For this review, take the finished solid that the model builds, in its own axes (mm). Coordinates: 2 decimals unless noted, no trailing zeros. Write each loop counter-clockwise with the first axis right and the second up, starting at its lowest first coordinate (ties: lowest second). Pieces come first, ordered by that corner, then holes. Notation, with made-up numbers: (58, 25.5) -> (115, 25.5) arc R19 ccw to (115, 33.5) -> close; hole circle Ø9 at (34.25, 0.5). An arc over 180 degrees is marked (long way). One line per item, written item: value. Start each with the question number.
1) For probe 1 along Z at (x, y) = (-9.6, -24.5); probe 2 along Y at (x, z) = (-9.4, 8.5); probe 3 along Y at (x, z) = (-10.65, 10), list the stretches that pass through material, from the lowest coordinate up. Write a range as from..to.
2) Add section C-C (z = 20). State the section outline as (x, y) points, and give its area (3 significant figures).
3) For pin 1 Ø1.5 at (y, z) = (-31, 32.5) entering from +X; pin 2 Ø1 at (x, z) = (-10, 32.5) entering from -Y; pin 3 Ø1 at (x, y) = (-10, -31.5) entering from +Z, all flat-tipped, find the tip position at first contact; note any pin that passes through.
4) Add section A-A (x = -10.1). State the section outline as (y, z) points.
5) Add section B-B (y = -66.5). State the section outline as (x, z) points, and give its area (3 significant figures).
Autodesk Inventor part; units mm, degrees
ref_plane "YZ Plane" through (0, 0, 0) normal (1, 0, 0) x (0, 1, 0)
ref_plane "XZ Plane" through (0, 0, 0) normal (0, 1, 0) x (-1, 0, 0)
ref_plane "XY Plane" through (0, 0, 0) normal (0, 0, 1) x (1, 0, 0)
ref_plane "Work Plane4" through (-12.2663, 34.5, -3) normal (-1, 0, 0) x (0, 0, 1)
sketch "Sketch4" plane through (-12.2663, 34.5, -3) normal (-1, 0, 0) x (0, 0, 1)
  line L0 (0, 0) -> (0, -108)
  line L1 (0, -108) -> (3, -108)
  line L2 (3, 0) -> (3, -108)
  line L3 (0, 0) -> (3, 0)
  circle A0 centre (13.5, 27.5) radius 25
  line L4 (7.5, -120) -> (3, -120)
  line L5 (3, -120) -> (3, -124)
  line L6 (3, -124) -> (-0.5, -124)
  line L7 (-0.5, -124) -> (-0.5, -138)
  line L8 (-0.5, -138) -> (8.5, -124)
  line L9 (8.5, -124) -> (7.5, -124)
  line L10 (7.5, -124) -> (7.5, -120)
  line L11 (0, -111) -> (3, -111)
  line L12 (0, -111) -> (0, -124)
  line L13 (0, -124) -> (3, -124)
  line L14 (3, -111) -> (3, -124)
  line L15 (3, -111) -> (3, -108)
  line L16 (0, -108) -> (0, -111)
  line L17 (7.5, -120) -> (3, -120)
  line L18 (3, -120) -> (3, 0)
  line L19 (3, 0) -> (36.5, 0)
  line L20 (8.5, -124) -> (66.1149, -34.3768)
  line L21 (7.5, -120) -> (63.7229, -32.5421)
  line L22 (36.5, 0) -> (36.5, -74.8889)
  line L23 (36.5, -72.0889) -> (33.5, -72.0889)
  line L24 (33.5, -72.0889) -> (33.5, -56.9889)
  line L25 (33.5, -56.9889) -> (36.5, -56.9889)
  line L26 (36.5, -56.9889) -> (36.5, -72.0889)
  point P0 (3, -34.5)
  point P1 (38.5, 27.5)
  point P2 (36.5, -56.9889)
  dimension "d4" = 25
  dimension "d5" = 2
  dimension "d9" = 2.8
  dimension "d10" = 15.1
  dimension "d11" = 3
extrude "Extrusion1" add sketch "Sketch4" against normal blind 3 contours L19 L22 L25 L24 L23 L21 L4 L14 L15 L2
sketch "Sketch8" plane through (-12.2663, -37.5889, 30.5) normal (0, 0, 1) x (1, 0, 0)
  line L0 (22.5, 14.9) -> (2, 14.9)
  line L1 (1.9, 14.8) -> (1.9, 0.3)
  line L2 (2, 0.2) -> (22.5, 0.2)
  line L3 (0, 0) -> (0, 15.1)
  line L4 (0, 0) -> (3, 0)
  line L5 (3, 15.1) -> (3, 0)
  line L6 (0, 15.1) -> (3, 15.1)
  line L7 (0, -2.8) -> (0, 0)
  line L8 (0, -2.8) -> (3, -2.8)
  line L9 (3, 0) -> (3, -2.8)
  line L10 (0, 0) -> (3, 0)
  line L11 (0, 15.1) -> (0, 72.0889)
  line L12 (0, 15.1) -> (3, 15.1)
  line L13 (3, 72.0889) -> (3, 15.1)
  line L14 (0, 72.0889) -> (3, 72.0889)
  line L15 (0, 15.1) -> (1.7, 15.1)
  line L16 (1.7, 15.1) -> (1.7, 0)
  line L17 (1.7, 0) -> (0, 0)
  line L18 (0, 0) -> (0, 15.1)
  point P0 (12.2663, 37.5889)
  point P1 (1.7, 0)
  point P2 (1.7, 15.1)
  dimension "d12" = 0.2
extrude "Extrusion2" add sketch "Sketch8" along normal up to surface (3 mm away) contours L3 L6 L16 L4
properties part number "right_side"
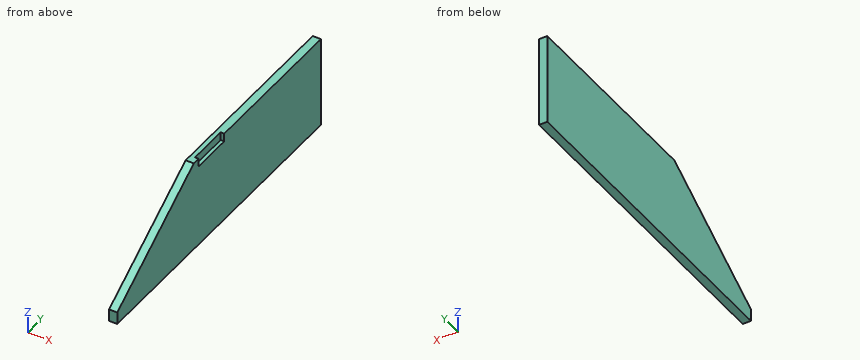
Numbers:
1. probe 1: 0..30.5
1. probe 2: -79.28..34.5
1. probe 3: -76.94..34.5
2. outline: (-12.27, -61.39) -> (-9.27, -61.39) -> (-9.27, 34.5) -> (-12.27, 34.5) -> close
2. area: 288 mm²
3. pin 1: x = -10.57
3. pin 2: y = -42.72
3. pin 3: z = 30.5
4. outline: (-85.5, 0) -> (34.5, 0) -> (34.5, 33.5) -> (-22.49, 33.5) -> (-22.49, 30.5) -> (-37.59, 30.5) -> (-37.59, 33.5) -> (-40.39, 33.5) -> (-85.5, 4.5) -> close
5. outline: (-12.27, 0) -> (-9.27, 0) -> (-9.27, 16.71) -> (-12.27, 16.71) -> close
5. area: 50.1 mm²
